from build123d import *

# Parameters (mm, degrees)
BOSS_EXTRUDE1_DEPTH      = 50
BOSS_EXTRUDE1_DEPTH_BACK = 30
SKETCH1_R                = 25


with BuildPart() as part:
    # Sketch1 → Boss-Extrude1 (new, two sides: drawn at the far end of the back side and taken through both)
    with BuildSketch(Plane(origin=(0, 0, 0), x_dir=(1, 0, 0), z_dir=(0, 1, 0)).offset(-BOSS_EXTRUDE1_DEPTH_BACK)):
        with Locations(Location((0, 0, 0), (0, 0, 270))):
            Circle(SKETCH1_R)
    extrude(amount=BOSS_EXTRUDE1_DEPTH + BOSS_EXTRUDE1_DEPTH_BACK)

    # Sketch3 → Cut-Revolve1 (revolve, cut)
    with BuildSketch(Plane.XY, mode=Mode.PRIVATE) as cut_revolve1_sk:
        Polygon((25, 0), (11.380324124, -30), (25, -30), align=None)
    revolve(cut_revolve1_sk.sketch.rotate(Axis((0, -30, 0), (0, 1, 0)), 90), axis=Axis((0, -30, 0), (0, 1, 0)), mode=Mode.SUBTRACT)

    # Sketch4 → Cut-Revolve2 (revolve, cut)
    with BuildSketch(Plane.XY, mode=Mode.PRIVATE) as cut_revolve2_sk:
        with BuildLine():
            Line((25, 41.301516329), (25, 10.643181842))
            ThreePointArc((25, 10.643181842), (21.760985667, 25.972349086), (25, 41.301516329))
        make_face()
    revolve(cut_revolve2_sk.sketch.rotate(Axis((0, -30, 0), (0, 1, 0)), 90), axis=Axis((0, -30, 0), (0, 1, 0)), mode=Mode.SUBTRACT)


solid = part.part
The listing builds one solid part. Answer for the finished solid, in the listing's coordinates (mm). Coordinates: 2 decimals unless noted, no trailing zeros. Order: outer loops, then holes, each group sorted by start corner. A loop starts at its lowest first (then second) coordinate and runs counter-clockwise, first axis right, second up.
Q1. Given P1, Ø1.5, axis at y = -10, z = 13, coming from the -X side; P2, Ø10, axis at x = -5.5, z = -17, coming from the -Y side; P3, Ø2, axis at y = 16.5, z = -0.5, coming from the +X side, each flat-ended and moving along its own axis, determine where each tip first touches the part or whether it passes through.
Q2. Consider line 1 (Y direction, x = -21.5, z = 11); line 2 (X direction, y = 41.5, z = 8.5); line 3 (X direction, y = 22, z = 13.5). Determine where each line is inside the solid, lowest interval first.
Q3. A cutting plane is placed at C-C, the plane y = -15.5. Write down the section's boundary in (x, z).
Q4. A cutting plane is placed at A-A, the plane x = 0. Write down the section's boundary in (y, z), and give its area (3 significant figures).
Q5. A cutting plane is placed at B-B, the plane z = 0. Write down the section's boundary in (x, y), and give its area (3 significant figures).
Answers follow:
1. P1: stops at x = -16.53
1. P2: stops at y = -26.72
1. P3: stops at x = 23.23
2. line 1: y = -1.87 to 12.73, 39.22 to 50
2. line 2: x = -23.51 to 23.51
2. line 3: x = -17.33 to 17.33
3. outline: circle Ø35.93 at (0, 0)
4. outline: (-30, -11.38) - (0, -25) - (10.64, -25) arc R37.89 cw to (41.3, -25) - (50, -25) - (50, 25) - (41.3, 25) arc R37.89 cw to (10.64, 25) - (0, 25) - (-30, 11.38) - close
4. area: 3,460 mm2
5. outline: (-25, 0) - (-11.38, -30) - (11.38, -30) - (25, 0) - (25, 10.64) arc R37.89 cw to (25, 41.3) - (25, 50) - (-25, 50) - (-25, 41.3) arc R37.89 cw to (-25, 10.64) - close
5. area: 3,460 mm2
